```python
from build123d import *

# Parameters (mm, degrees)
SKETCH1_R           = 25.4
SKETCH1_R_2         = 3.031432634
BOSS_EXTRUDE1_DEPTH = 6.35


with BuildPart() as part:
    # Sketch1 → Boss-Extrude1 (new body)
    with BuildSketch(Plane(origin=(0, 0, 0), x_dir=(0, 0, -1), z_dir=(1, 0, 0))):
        Circle(SKETCH1_R)
        Circle(SKETCH1_R_2, mode=Mode.SUBTRACT)
        with BuildLine():
            ThreePointArc((-12.796678201, 1.768771626), (-13.596470588, -14.067117647), (0, -22.225))
            ThreePointArc((0, -22.225), (3.175, -19.05), (0, -15.875))
            ThreePointArc((0, -15.875), (-7.993529412, -11.078882353), (-7.523321799, -1.768771626))
            ThreePointArc((-7.523321799, -1.768771626), (-8.391228374, 2.636678201), (-12.796678201, 1.768771626))
        make_face(mode=Mode.SUBTRACT)
    extrude(amount=BOSS_EXTRUDE1_DEPTH)


solid = part.part
```
The model under review builds one solid part; all positions refer to its coordinate system, in mm. A direction names the side the tool comes from. Round coordinates to 2 decimals unless told otherwise and drop trailing zeros. Loops run counter-clockwise (first coordinate to the right, second up) from the corner with the lowest first, then second, coordinate; pieces in that order, holes last.
1) Wall thickness on line 1 along Y through (x, z) = (2.75, 0) (3 decimals); line 2 along Y through (x, z) = (2.5, 7.5); line 3 along Y through (x, z) = (3.75, 5.5): over which ranges is each line inside the solid? List them lowest first.
Values follow:
line 1: y = -25.4 to -22.225, -15.875 to -3.031, 3.031 to 25.4
line 2: y = -24.27 to -20.28, -11.9 to -1.73, 1.73 to 24.27
line 3: y = -24.8 to -21.21, -14.01 to 24.8
2) The part is to be moulded in two halves that separate along Y. For faces 3 (the face through (3.131, -24.796, 5.506)), 4 (the face through (3.131, -19.12, -3.174)), 5 (the face through (0, 0, -5)), say which applies: pulls with the +Y half, pulls with the -Y half, needs draft (parallel to the pull), parting line crosses it, or undercut.
Values follow:
face 3: parting line crosses it
face 4: undercut
face 5: needs draft
3) Clearance check with flat-ended pins moving along their axes: P1, Ø3, axis at x = 4.5, z = -19.5, coming from the +Y side; P2, Ø1.5, axis at x = 3.5, z = -4.5, coming from the -Y side; P3, Ø1, axis at x = 3.5, y = 17, coming from the -Z side. State where each tip first meets the part, or that it passes through.
Values follow:
P1: stops at y = 17.92
P2: stops at y = -25.12
P3: stops at z = -19.31
4) Consider section D-D on x = 3.5. State the section outline as (y, z) points (3 decimals).
Values follow:
outline: circle Ø50.8 at (0, 0); hole (-22.225, 0) arc R3.175 ccw to (-15.875, 0) arc R9.059 cw to (-1.769, 7.523) arc R3.175 ccw to (1.769, 12.797) arc R15.409 ccw to start; hole circle Ø6.063 at (0, 0)
5) Consider section B-B on y = -1. State the section outline as (x, z) points, then the cut area to 3 significant figures.
Values follow:
outline: (0, -25.38) - (6.35, -25.38) - (6.35, -2.86) - (0, -2.86) - close; (0, 2.86) - (6.35, 2.86) - (6.35, 7.15) - (0, 7.15) - close; (0, 14.27) - (6.35, 14.27) - (6.35, 25.38) - (0, 25.38) - close
area: 241 mm2
6) Consider section A-A on z = 10.16. State the section outline as (x, y) points (3 decimals).
Values follow:
outline: (0, -23.279) - (6.35, -23.279) - (6.35, -18.401) - (0, -18.401) - close; (0, 3.175) - (6.35, 3.175) - (6.35, 23.279) - (0, 23.279) - close
7) Tool access review of faces 1 (the face through (3.13, -11.2, 7.93)), 2 (the face through (6.35, 0, -5)): name each direction out of +Z, -Z, +X, -X, +Y, -Y from which nothing blocks a thin tool from reaching the whole face with its end or side.
Values follow:
face 1: +X, -X
face 2: +Z, -Z, +X, +Y, -Y
